Design review of the part built by this model. Coordinates are the model's own, in mm. A direction names the side the tool comes from. Round coordinates to 2 decimals unless told otherwise and drop trailing zeros. Loops run counter-clockwise (first coordinate to the right, second up) from the corner with the lowest first, then second, coordinate; pieces in that order, holes last. Notation, with made-up numbers: M -35.75,19 L -3.75,19 A7 ccw -3.75,30 Z; hole C -33,-35.75 d3. An arc over 180 degrees is marked long. One line per item, written item: value. Start each with the question number.
Item 1: We need section C-C (z = -11.5). Write out the cut boundary in (x, y), then the cut area to 3 significant figures.
Item 2: Clearance check with flat-ended pins moving along their axes: pin 1 (10 mm diameter, centred on x = 165, y = 19.5, fed in from -Z); pin 2 (4.5 mm diameter, centred on y = -2, z = -17.5, fed in from -X); pin 3 (3 mm diameter, centred on y = -8, z = -46, fed in from -X); pin 4 (22.5 mm diameter, centred on x = -11, y = -6, fed in from -Z). State where each tip first meets the part, or that it passes through.
Item 3: Mouldability with a two-part tool opening along X and no side actions: class faces 1 (the flat face through (3, -30, -25)), 2 (the cylindrical face through (212.47, 1.32, -35.64)), 3 (the flat face through (-195, -13, -59)) as released by +X, released by -X, zero draft, split by the parting line, or undercut.
Item 4: We need section B-B (z = -71.5). Write out the cut boundary in (x, y).
Item 5: We need section D-D (y = 5.5). Write out the cut boundary in (x, z), then the cut area to 3 significant figures.
Item 6: For line 1 along Y through (x, z) = (0, -4.5); line 2 along Z through (x, y) = (-5, -25.5); line 3 along Z through (x, y) = (131.5, 16), list the stretches that pass through material, from the lowest coordinate up.
Item 7: We need section A-A (x = 0). Write out the cut boundary in (y, z), then the cut area to 3 significant figures.
Item 8: For faces 4 (the cylindrical face through (-166.104, -6.798, -81.924)), 5 (the flat face through (30, -8, -15)), 6 (the flat face through (-3, 30, -15)), list the 3-axis set-ups (+Z, -Z, +X, -X, +Y, -Y) from which the entire face can be reached by the end or side of a thin tool; tool diameter is ignored.
from build123d import *

# Parameters (mm, degrees)
BOSS_EXTRUDE1_DEPTH = 30
SKETCH2_R           = 30
BOSS_EXTRUDE2_DEPTH = 29
SKETCH1_3_R         = 10
CUT_EXTRUDE1_DEPTH  = 30
BOSS_EXTRUDE3_START = -59
SKETCH1_4_R         = 17.75
BOSS_EXTRUDE3_DEPTH = 46.5
SKETCH3_W           = 60
SKETCH3_H           = 15
CUT_EXTRUDE2_DEPTH  = 45


with BuildPart() as part:
    # Sketch1 → Boss-Extrude1 (new body)
    with BuildSketch(Plane.XY):
        with BuildLine():
            Line((-182.5, 30), (182.5, 30))
            ThreePointArc((182.5, 30), (212.5, 0), (182.5, -30))
            Line((182.5, -30), (-182.5, -30))
            ThreePointArc((-182.5, -30), (-212.5, 0), (-182.5, 30))
        make_face()
    extrude(amount=-BOSS_EXTRUDE1_DEPTH)

    # Sketch2 → Boss-Extrude2 (add)
    with BuildSketch(Plane(origin=(0, 0, -30), x_dir=(-1, 0, 0), z_dir=(0, 0, -1))):
        with Locations((-182.5, 0)):
            Circle(SKETCH2_R)
        with Locations((182.5, 0)):
            Circle(SKETCH2_R)
    extrude(amount=BOSS_EXTRUDE2_DEPTH)

    # Sketch1<3> → Cut-Extrude1 (cut)
    with BuildSketch(Plane.XY):
        Circle(SKETCH1_3_R)
    extrude(amount=-CUT_EXTRUDE1_DEPTH, mode=Mode.SUBTRACT)

    # Sketch1<4> → Boss-Extrude3 (add)
    with BuildSketch(Plane.XY.offset(BOSS_EXTRUDE3_START)):
        with Locations((182.5, 0)):
            Circle(SKETCH1_4_R)
        with Locations((-182.5, 0)):
            Circle(SKETCH1_4_R)
    extrude(amount=-BOSS_EXTRUDE3_DEPTH)

    # Sketch3 → Cut-Extrude2 (cut)
    with BuildSketch(Plane.XZ.offset(30)):
        with Locations((0, -15)):
            Rectangle(SKETCH3_W, SKETCH3_H)
    extrude(amount=-CUT_EXTRUDE2_DEPTH, mode=Mode.SUBTRACT)


solid = part.part
A:
1. outline: M -182.5,-30 L -30,-30 L -30,15 L 30,15 L 30,-30 L 182.5,-30 A30 ccw 182.5,30 L -182.5,30 A30 ccw Z
1. area: 22,000 mm2
2. pin 1: z = -59
2. pin 2: x = -212.5
2. pin 3: x = -211.79
2. pin 4: z = -30
3. face 1: zero draft
3. face 2: undercut
3. face 3: undercut
4. outline: C -182.5,0 d35.5; C 182.5,0 d35.5
5. outline: M -211.99,-59 L -199.38,-59 L -199.38,-105.5 L -165.62,-105.5 L -165.62,-59 L -153.01,-59 L -153.01,-30 L -8.35,-30 L -8.35,-22.5 L -30,-22.5 L -30,-7.5 L -8.35,-7.5 L -8.35,0 L -211.99,0 Z; M 8.35,-30 L 153.01,-30 L 153.01,-59 L 165.62,-59 L 165.62,-105.5 L 199.38,-105.5 L 199.38,-59 L 211.99,-59 L 211.99,0 L 8.35,0 L 8.35,-7.5 L 30,-7.5 L 30,-22.5 L 8.35,-22.5 Z
5. area: 18,100 mm2
6. line 1: -30 to -10, 10 to 30
6. line 2: -30 to -22.5, -7.5 to 0
6. line 3: -30 to 0
7. outline: M -30,-30 L -10,-30 L -10,-22.5 L -30,-22.5 Z; M -30,-7.5 L -10,-7.5 L -10,0 L -30,0 Z; M 10,-30 L 30,-30 L 30,0 L 10,0 L 10,-7.5 L 15,-7.5 L 15,-22.5 L 10,-22.5 Z
7. area: 825 mm2
8. face 4: -Z
8. face 5: -Y
8. face 6: +Z, -Z, +X, -X, +Y
